Can you work these out from the model? Positions are in its coordinate system, mm. A direction names the side the tool comes from. Round coordinates to 2 decimals unless told otherwise and drop trailing zeros. Order: outer loops, then holes, each group sorted by start corner. A loop starts at its lowest first (then second) coordinate and runs counter-clockwise, first axis right, second up.
Q1. If I drill on line 1 (Z direction, x = -0.5, y = -0.45); line 2 (X direction, y = -1.9, z = -1.75); line 3 (Y direction, x = -1.5, z = -2), over which ranges is the centre line in solid material (lowest first)?
Q2. If we section it at A-A (y = -0.8): Please give me the cut outline in (x, z).
Q3. Will these pins go through, and if not, where does the flat tip stop? P1, Ø0.6, axis at x = -0.5, z = -6, coming from the -Y side; P2, Ø0.6, axis at x = -2.5, z = 4, coming from the -Y side; P3, Ø0.6, axis at x = -2.5, z = -4, coming from the +Y side.
Q4. If we section it at D-D (y = -1.8): Please give me the cut outline in (x, z), plus the area to 3 significant figures.
Q5. For faces 5 (the face through (-1.6, -1.5, 0)), 6 (the face through (-1, -0.5, -5.5)), 7 (the face through (0, -1, -5)), which set-ups out of +Z, -Z, +X, -X, +Y, -Y let a thin tool reach every point of the face, with its end or its side?
Q6. If we section it at C-C (z = 0): Please give me the cut outline in (x, y).
Q7. We'd pull the mould along Z, two halves only. Please class faces 1 (the face through (0, 1, 0)), 2 (the face through (0, -1, 4)), 3 (the face through (0, -1, -4)), 4 (the face through (0, 0, 4.5)): pulls with the +Z half, pulls with the -Z half, needs draft (parallel to the pull), parting line crosses it, or undercut.
Q8. If we section it at B-B (x = 1.75): Please give me the cut outline in (y, z).
from build123d import *

# Parameters (mm, degrees)
SKETCH_1_W      = 4
SKETCH_1_H      = 8
EXTRUDE_1_DEPTH = 1
SKETCH_2_W      = 4
SKETCH_2_H      = 2.5
EXTRUDE_2_DEPTH = 0.5
SKETCH_3_W      = 4
SKETCH_3_H      = 9
SKETCH_3_W_2    = 2.8
SKETCH_3_H_2    = 7.8
EXTRUDE_3_DEPTH = 0.5
EXTRUDE_4_DEPTH = 0.5
SKETCH_5_W      = 2
SKETCH_5_H      = 1
EXTRUDE_5_DEPTH = 2


with BuildPart() as part:
    # 草图1 → 凸台-拉伸1 (new body)
    with BuildSketch(Plane(origin=(0, 0, 0), x_dir=(1, 0, 0), z_dir=(0, 1, 0))):
        Rectangle(SKETCH_1_W, SKETCH_1_H)
    extrude(amount=EXTRUDE_1_DEPTH)

    # 草图2 → 凸台-拉伸2 (add)
    with BuildSketch(Plane(origin=(0, 0, -4), x_dir=(-1, 0, 0), z_dir=(0, 0, -1))):
        with Locations((0, -0.25)):
            Rectangle(SKETCH_2_W, SKETCH_2_H)
    extrude_2 = extrude(amount=EXTRUDE_2_DEPTH)

    # 镜向1: 凸台-拉伸2 across plane
    add(extrude_2.mirror(Plane.XY))

    # 草图3 → 凸台-拉伸3 (add)
    with BuildSketch(Plane.XZ.offset(1.5)):
        Rectangle(SKETCH_3_W, SKETCH_3_H)
        Rectangle(SKETCH_3_W_2, SKETCH_3_H_2, mode=Mode.SUBTRACT)
    extrude(amount=EXTRUDE_3_DEPTH)

    # 草图4 → 凸台-拉伸4 (add)
    with BuildSketch(Plane(origin=(0, 0, 0), x_dir=(1, 0, 0), z_dir=(0, 1, 0))):
        with BuildLine():
            Line((-2, 4.5), (-3.138641266, 4.5))
            ThreePointArc((-3.138641266, 4.5), (-2.791797675, 4.020569497), (-2.227919338, 4.2))
            Line((-2.227919338, 4.2), (2.227919338, 4.2))
            ThreePointArc((2.227919338, 4.2), (2.791797675, 4.020569497), (3.138641266, 4.5))
            Line((3.138641266, 4.5), (2, 4.5))
            Line((2, 4.5), (-2, 4.5))
        make_face()
        with BuildLine():
            Line((2, -4.5), (3.138641266, -4.5))
            ThreePointArc((3.138641266, -4.5), (2.791797675, -4.020569497), (2.227919338, -4.2))
            Line((2.227919338, -4.2), (-2.227919338, -4.2))
            ThreePointArc((-2.227919338, -4.2), (-2.791797675, -4.020569497), (-3.138641266, -4.5))
            Line((-3.138641266, -4.5), (-2, -4.5))
            Line((-2, -4.5), (2, -4.5))
        make_face()
    extrude(amount=-EXTRUDE_4_DEPTH)

    # 草图5 → 凸台-拉伸5 (add)
    with BuildSketch(Plane(origin=(0, 0, -4.5), x_dir=(-1, 0, 0), z_dir=(0, 0, -1))):
        with Locations((0, -0.5)):
            Rectangle(SKETCH_5_W, SKETCH_5_H)
    extrude(amount=EXTRUDE_5_DEPTH)


solid = part.part
Solution:
1. line 1: z = -6.5 to -4, 4 to 4.5
1. line 2: x = -2 to -1.4, 1.4 to 2
1. line 3: y = -2 to -1.5, 0 to 1
2. outline: (-2, -4.5) - (-1, -4.5) - (-1, -6.5) - (1, -6.5) - (1, -4.5) - (2, -4.5) - (2, -4) - (-2, -4) - close; (-2, 4) - (2, 4) - (2, 4.5) - (-2, 4.5) - close
3. P1: stops at y = -1
3. P2: stops at y = -0.5
3. P3: stops at y = 0
4. outline: (-2, -4.5) - (2, -4.5) - (2, 4.5) - (-2, 4.5) - close; hole (-1.4, -3.9) - (1.4, -3.9) - (1.4, 3.9) - (-1.4, 3.9) - close
4. area: 14.2 mm2
5. face 5: +X, -X
5. face 6: -Z, -X, +Y, -Y
5. face 7: -Z, +X, -X, -Y
6. outline: (-2, -2) - (-1.4, -2) - (-1.4, -1.5) - (-2, -1.5) - close; (-2, 0) - (2, 0) - (2, 1) - (-2, 1) - close; (1.4, -2) - (2, -2) - (2, -1.5) - (1.4, -1.5) - close
7. face 1: needs draft
7. face 2: undercut
7. face 3: undercut
7. face 4: pulls with the +Z half
8. outline: (-2, -4.5) - (1, -4.5) - (1, 4.5) - (-2, 4.5) - close; hole (-1.5, -4) - (0, -4) - (0, 4) - (-1.5, 4) - close
